Read the model definition and answer for the solid it produces. Units are mm, in the model's axes. A direction names the side the tool comes from. Round coordinates to 2 decimals unless told otherwise and drop trailing zeros. Write each loop counter-clockwise with the first axis right and the second up, starting at its lowest first coordinate (ties: lowest second). Pieces come first, ordered by that corner, then holes. Notation, with made-up numbers: (44.5, -10) -> (75.5, -10) arc R4 ccw to (75.5, -4) -> close; hole circle Ø6 at (-1, -39). An arc over 180 degrees is marked (long way). Return JSON: item names as keys, results as strings.
from build123d import *

# Parameters (mm, degrees)
SKETCH1_R           = 3.9
SKETCH1_R_2         = 2.48
BOSS_EXTRUDE1_DEPTH = 16
CUT_EXTRUDE1_START  = -0.93
SKETCH2_R           = 3.14
SKETCH2_R_2         = 2.48
CUT_EXTRUDE1_DEPTH  = 0.93
SKETCH3_R           = 3.14
SKETCH3_R_2         = 2.48
CUT_EXTRUDE3_DEPTH  = 0.93
SKETCH4_R           = 0.93
WRAP1_START         = 1.46
WRAP1_DEPTH         = 0.1
WRAP1_START_2       = 14.44
WRAP1_2_DEPTH       = 0.1


# Read off the part's stored shape, not the designer's step: Wrap1
with BuildPart() as part:
    # Sketch1 → Boss-Extrude1 (new body)
    with BuildSketch(Plane.XY):
        Circle(SKETCH1_R)
        Circle(SKETCH1_R_2, mode=Mode.SUBTRACT)
    extrude(amount=BOSS_EXTRUDE1_DEPTH)

    # Sketch2 → Cut-Extrude1 (cut)
    with BuildSketch(Plane.XY.offset(16).offset(CUT_EXTRUDE1_START)):
        Circle(SKETCH2_R)
        Circle(SKETCH2_R_2, mode=Mode.SUBTRACT)
    extrude(amount=CUT_EXTRUDE1_DEPTH, mode=Mode.SUBTRACT)

    # Sketch3 → Cut-Extrude3 (cut)
    with BuildSketch(Plane.XY):
        Circle(SKETCH3_R)
        Circle(SKETCH3_R_2, mode=Mode.SUBTRACT)
    extrude(amount=CUT_EXTRUDE3_DEPTH, mode=Mode.SUBTRACT)

    # Sketch4 → Cut-Revolve1 (revolve, cut)
    with BuildSketch(Plane(origin=(0, 0, 0), x_dir=(1, 0, 0), z_dir=(0, 1, 0)), mode=Mode.PRIVATE) as cut_revolve1_sk:
        with Locations((2.48, -8)):
            Circle(SKETCH4_R)
    revolve(cut_revolve1_sk.sketch.rotate(Axis((0, 0, 0.93), (0, 0, 1)), 180), axis=Axis((0, 0, 0.93), (0, 0, 1)), mode=Mode.SUBTRACT)

    # Wrap1 outline → Wrap1 (cut)
    with BuildSketch(Plane.XY.offset(WRAP1_START)):
        with BuildLine():
            Line((-2.107178993, -3.281736841), (-2.080163878, -3.239663292))
            ThreePointArc((-2.080163878, -3.239663292), (2.078325496, 3.240842967), (-2.076488681, -3.242020166))
            Line((-2.076488681, -3.242020166), (-2.103456067, -3.284124324))
            ThreePointArc((-2.103456067, -3.284124324), (2.105317868, 3.28293111), (-2.107178993, -3.281736841))
        make_face()
    extrude(amount=WRAP1_DEPTH, mode=Mode.SUBTRACT)

    # Wrap1 2 outline → Wrap1 2 (cut)
    with BuildSketch(Plane.XY.offset(WRAP1_START_2)):
        with BuildLine():
            Line((-2.107178993, -3.281736841), (-2.080163878, -3.239663292))
            ThreePointArc((-2.080163878, -3.239663292), (2.078325496, 3.240842967), (-2.076488681, -3.242020166))
            Line((-2.076488681, -3.242020166), (-2.103456067, -3.284124324))
            ThreePointArc((-2.103456067, -3.284124324), (2.105317868, 3.28293111), (-2.107178993, -3.281736841))
        make_face()
    extrude(amount=WRAP1_2_DEPTH, mode=Mode.SUBTRACT)


solid = part.part
Item 1: Straight lines are drawn through the part: L1, parallel to Y at x = 0, z = 15.85; L2, parallel to Y at x = 0, z = 4.25; L3, parallel to X at y = 1.5, z = 14.5. For each, find the intervals that lie inside material, in ascending order. Write a range as [from, to].
Worked answers:
{"L1": "y = [-3.9, -3.14], [3.14, 3.9]", "L2": "y = [-3.9, -2.48], [2.48, 3.9]", "L3": "x = [-3.55, -1.97], [1.97, 3.55]"}
Item 2: A tool of negligible diameter and unlimited length cuts with its end or side. For faces 1 (the cylindrical face through (2.995, 0.943, 0.458)), 2 (the flat face through (-3, 2, 16)), 3 (the cylindrical face through (2.995, 0.943, 15.528)), from which of +Z, -Z, +X, -X, +Y, -Y can it reach the whole face along a straight path? Write none if from no direction.
Worked answers:
{"face 1": "-Z", "face 2": "+Z, +X, -X, +Y, -Y", "face 3": "+Z"}
Item 3: Section A-A (z = 11) is taken. Give the vertices of the cut face in (x, y), then the cut area to 3 significant figures.
Worked answers:
{"outline": "circle Ø7.8 at (0, 0); hole circle Ø4.96 at (0, 0)", "area": "28.5 mm2"}
Item 4: Flat-ended cylindrical pins translate along their axes: pin 1 (4 mm diameter, centred on x = 0, y = 0, fed in from -Z); pin 2 (1 mm diameter, centred on x = -2.5, z = 9.5, fed in from +Y); pin 3 (3 mm diameter, centred on x = -1, y = 1, fed in from -Z); pin 4 (1 mm diameter, centred on y = -2, z = 2.5, fed in from -X). Find the tip coordinate at first contact, or state that the pin passes through.
Worked answers:
{"pin 1": "passes through", "pin 2": "stops at y = 3.35", "pin 3": "stops at z = 0.93", "pin 4": "stops at x = -3.6"}
